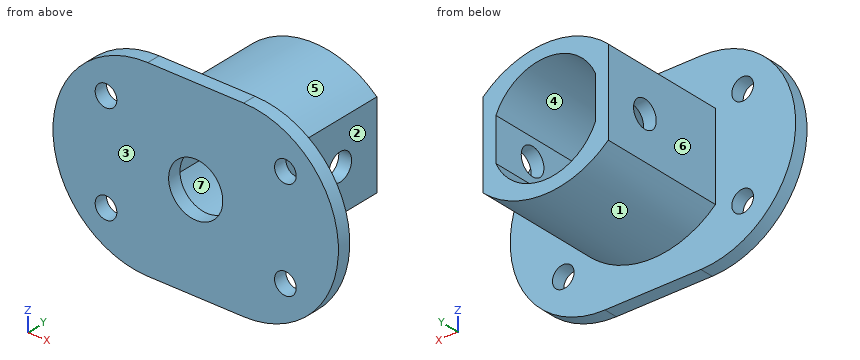
from build123d import *

# Parameters (mm, degrees)
BOSS_EXTRUDE1_DEPTH = 3.175
SKETCH2_R           = 2.54
CUT_EXTRUDE1_DEPTH  = 41.306412331
BOSS_EXTRUDE2_DEPTH = 30
SKETCH4_R           = 6.35
CUT_EXTRUDE2_DEPTH  = 51.145052099
SKETCH6_R           = 3.175
CUT_EXTRUDE3_DEPTH  = 66.447021029


with BuildPart() as part:
    # Sketch1 → Boss-Extrude1 (new body)
    with BuildSketch(Plane(origin=(0, 0, 0), x_dir=(1, 0, 0), z_dir=(0, 1, 0))):
        with BuildLine():
            Line((-11.25, 22.225), (11.25, 22.225))
            ThreePointArc((11.25, 22.225), (33.475, 0), (11.25, -22.225))
            Line((11.25, -22.225), (-11.25, -22.225))
            ThreePointArc((-11.25, -22.225), (-33.475, 0), (-11.25, 22.225))
        make_face()
    extrude(amount=BOSS_EXTRUDE1_DEPTH)

    # Sketch2 → Cut-Extrude1 (cut, through all)
    with BuildSketch(Plane(origin=(0, 3.175, 0), x_dir=(1, 0, 0), z_dir=(0, 1, 0))):
        with Locations(Location((-21.036441357, -11.663026646, 0), (0, 0, 270))):
            Circle(SKETCH2_R)
        with Locations(Location((-21.036441357, 11.663026646, 0), (0, 0, 270))):
            Circle(SKETCH2_R)
        with Locations(Location((21.036441357, -11.663026646, 0), (0, 0, 90))):
            Circle(SKETCH2_R)
        with Locations(Location((21.036441357, 11.663026646, 0), (0, 0, 90))):
            Circle(SKETCH2_R)
    extrude(amount=-CUT_EXTRUDE1_DEPTH, mode=Mode.SUBTRACT)

    # Sketch3 → Boss-Extrude2 (add)
    with BuildSketch(Plane(origin=(0, 3.175, 0), x_dir=(1, 0, 0), z_dir=(0, 1, 0))):
        with BuildLine():
            Line((-14.674330816, -10), (-14.674330816, 10))
            ThreePointArc((-14.674330816, 10), (0, 15.7), (14.674330816, 10))
            Line((14.674330816, 10), (14.674330816, -10))
            ThreePointArc((14.674330816, -10), (0, -15.7), (-14.674330816, -10))
        make_face()
        with BuildLine():
            Line((-11.674330816, 5), (-11.674330816, -5))
            ThreePointArc((-11.674330816, -5), (0, -12.7), (11.674330816, -5))
            Line((11.674330816, -5), (11.674330816, 5))
            ThreePointArc((11.674330816, 5), (0, 12.7), (-11.674330816, 5))
        make_face(mode=Mode.SUBTRACT)
    extrude(amount=BOSS_EXTRUDE2_DEPTH)

    # Sketch4 → Cut-Extrude2 (cut, through all)
    with BuildSketch(Plane(origin=(0, 3.175, 0), x_dir=(1, 0, 0), z_dir=(0, 1, 0))):
        with Locations(Location((0, 0, 0), (0, 0, 270))):
            Circle(SKETCH4_R)
    extrude(amount=-CUT_EXTRUDE2_DEPTH, mode=Mode.SUBTRACT)

    # Sketch6 → Cut-Extrude3 (cut, through all)
    with BuildSketch(Plane(origin=(-14.674330816, 2.247424982, 9.530938138), x_dir=(0, 0, 1), z_dir=(-1, 0, 0))):
        with Locations((-9.530938138, 20.677575018)):
            Circle(SKETCH6_R)
    extrude(amount=-CUT_EXTRUDE3_DEPTH, mode=Mode.SUBTRACT)


solid = part.part
Verification items for the finished model (mm, model axes). Face numbers are marked on the shaded views. A direction names the side the tool comes from. Coordinates: 2 decimals unless noted, no trailing zeros. Order: outer loops, then holes, each group sorted by start corner. A loop starts at its lowest first (then second) coordinate and runs counter-clockwise, first axis right, second up. Notation, with made-up numbers: M 76.5,42 L 123.5,42 A18 cw 123.5,74 Z; hole C 66.5,-37.75 d10. An arc over 180 degrees is marked long. One line per item, written item: value. Start each with the question number.
Item 1: Mould release check, pull along Z, two halves, no side actions. Record for the marked faces 5, 6 and 7: released by +Z, released by -Z, zero draft, split by the parting line, or undercut.
Item 2: Access from +Z, -Z, +X, -X, +Y, -Y to the whole of each face (thin tool, end or side, straight path). Record for the marked faces 1, 2, 3 and 4.
Item 3: Gauge pin test, flat ends, axial feed: pin 1 (3 mm diameter, centred on y = 29, z = 8.5, fed in from -X); pin 2 (3 mm diameter, centred on y = 11.5, z = 2.5, fed in from +X); pin 3 (11.5 mm diameter, centred on x = 2, z = 5.5, fed in from +Y) (3 decimals). Record the tip position at first contact, or that the pin passes through.
Item 4: Scan lines: probe 1 along X at (y, z) = (3.5, 4); probe 2 along X at (y, z) = (1.65, 0) (3 decimals); probe 3 along Y at (x, z) = (-18, -5) (3 decimals). Record each from-to range of solid material in increasing order.
Item 5: Sectioned sample at D-D (x = 24.5). Enter the section's corners in (y, z) (3 decimals), then the cut area to 3 significant figures.
Item 6: Sectioned sample at A-A (z = 0). Enter the section's corners in (x, y) (3 decimals), then the cut area to 3 significant figures.
Item 7: Sectioned sample at B-B (x = 0). Enter the section's corners in (y, z) (3 decimals), then the cut area to 3 significant figures.
Item 8: Sectioned sample at C-C (y = 22). Enter the section's corners in (x, z), then the cut area to 3 significant figures.
Conclusion:
1. face 5: released by +Z
1. face 6: zero draft
1. face 7: undercut
2. face 1: -Z, +Y
2. face 2: +Z, -Z, +X, +Y
2. face 3: +Z, -Z, +X, -X, -Y
2. face 4: +Y
3. pin 1: stops at x = -14.67
3. pin 2: stops at x = 14.67
3. pin 3: stops at y = 3.175
4. probe 1: x = -14.67 to -11.67, 11.67 to 14.67
4. probe 2: x = -33.475 to -6.35, 6.35 to 33.475
4. probe 3: y = 0 to 3.175
5. outline: M 0,-17.843 L 3.175,-17.843 L 3.175,17.843 L 0,17.843 Z
5. area: 113 mm^2
6. outline: M -33.475,0 L -6.35,0 L -6.35,3.175 L -11.674,3.175 L -11.674,19.75 L -14.674,19.75 L -14.674,3.175 L -33.475,3.175 Z; M -14.674,26.1 L -11.674,26.1 L -11.674,33.175 L -14.674,33.175 Z; M 6.35,0 L 33.475,0 L 33.475,3.175 L 14.674,3.175 L 14.674,19.75 L 11.674,19.75 L 11.674,3.175 L 6.35,3.175 Z; M 11.674,26.1 L 14.674,26.1 L 14.674,33.175 L 11.674,33.175 Z
6. area: 314 mm^2
7. outline: M 0,-22.225 L 3.175,-22.225 L 3.175,-15.7 L 33.175,-15.7 L 33.175,-12.7 L 3.175,-12.7 L 3.175,-6.35 L 0,-6.35 Z; M 0,6.35 L 3.175,6.35 L 3.175,12.7 L 33.175,12.7 L 33.175,15.7 L 3.175,15.7 L 3.175,22.225 L 0,22.225 Z
7. area: 281 mm^2
8. outline: M -14.67,-10 A21.74 ccw 14.67,-10 L 14.67,-3.04 L 11.67,-3.04 L 11.67,-5 A12.7 cw -11.67,-5 L -11.67,-3.04 L -14.67,-3.04 Z; M -14.67,3.04 L -11.67,3.04 L -11.67,5 A12.7 cw 11.67,5 L 11.67,3.04 L 14.67,3.04 L 14.67,10 A21.74 ccw -14.67,10 Z
8. area: 287 mm^2
